The figure shows three views and two pictorial views of one solid part (mm, origin at its lowest corner). Answer the questions. Coordinates: 2 decimals unless noted, no trailing zeros. Write each loop counter-clockwise with the first axis right and the second up, starting at its lowest first coordinate (ties: lowest second). Pieces come first, ordered by that corner, then holes. Notation, with made-up numbers: M 23.25,18 L 30.25,18 A7 ccw 30.25,25 Z; hole C 75.25,-9.75 d1. An arc over 180 degrees is marked long. Use CSV: the item, a comma, the result in double quotes.
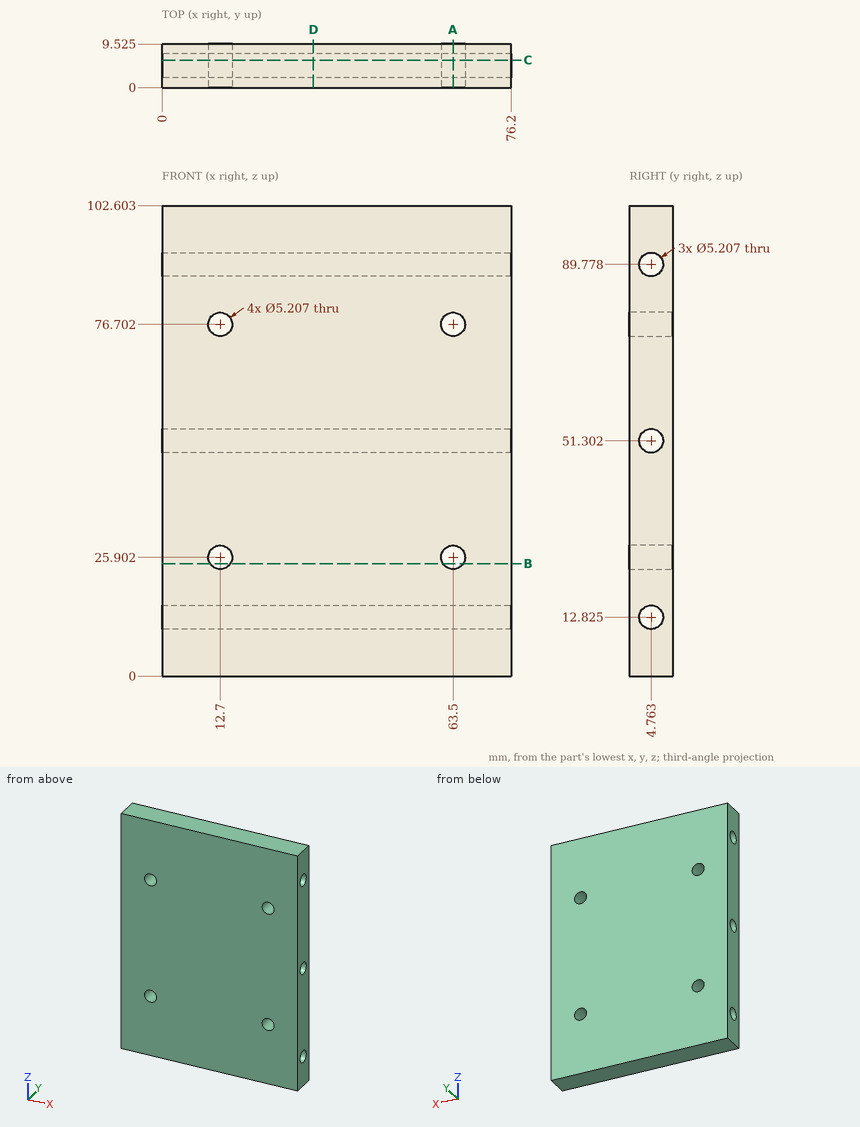
Item 1: The part is cut by section B-B (z = 24.5). Write down the section's boundary in (x, y) (1 decimal).
Answer:
outline,"M 0,0 L 10.5,0 L 10.5,9.5 L 0,9.5 Z; M 14.9,0 L 61.3,0 L 61.3,9.5 L 14.9,9.5 Z; M 65.7,0 L 76.2,0 L 76.2,9.5 L 65.7,9.5 Z"
Item 2: The part is cut by section C-C (y = 6). Write down the section's boundary in (x, z) (1 decimal), then the cut area to 3 significant figures.
Answer:
outline,"M 0,0 L 76.2,0 L 76.2,10.5 L 0,10.5 Z; M 0,15.1 L 76.2,15.1 L 76.2,49 L 0,49 Z; M 0,53.6 L 76.2,53.6 L 76.2,87.5 L 0,87.5 Z; M 0,92.1 L 76.2,92.1 L 76.2,102.6 L 0,102.6 Z; hole C 12.7,25.9 d5.2; hole C 12.7,76.7 d5.2; hole C 63.5,25.9 d5.2; hole C 63.5,76.7 d5.2"
area,"6,690 mm2"
Item 3: Consider probe 1 along Z at (x, y) = (63.5, 4.5) (1 decimal); probe 2 along X at (y, z) = (2.75, 77.5); probe 3 along Z at (x, y) = (52.5, 2.5) (1 decimal). Determine where each line is inside the solid, lowest interval first.
Answer:
probe 1,"z = 0 to 10.2, 15.4 to 23.3, 28.5 to 48.7, 53.9 to 74.1, 79.3 to 87.2, 92.4 to 102.6"
probe 2,"x = 0 to 10.22, 15.18 to 61.02, 65.98 to 76.2"
probe 3,"z = 0 to 11.5, 14.1 to 50, 52.6 to 88.5, 91.1 to 102.6"
Item 4: The part is cut by section D-D (x = 33). Write down the section's boundary in (y, z) (1 decimal).
Answer:
outline,"M 0,0 L 9.5,0 L 9.5,102.6 L 0,102.6 Z; hole C 4.8,12.8 d5.2; hole C 4.8,51.3 d5.2; hole C 4.8,89.8 d5.2"
Item 5: The part is cut by section A-A (x = 63.5). Write down the section's boundary in (y, z) (1 decimal).
Answer:
outline,"M 0,0 L 9.5,0 L 9.5,23.3 L 0,23.3 Z; M 0,28.5 L 9.5,28.5 L 9.5,74.1 L 0,74.1 Z; M 0,79.3 L 9.5,79.3 L 9.5,102.6 L 0,102.6 Z; hole C 4.8,12.8 d5.2; hole C 4.8,51.3 d5.2; hole C 4.8,89.8 d5.2"
